Verification items for the finished model (mm, model axes). Face numbers are marked on the shaded views. A direction names the side the tool comes from. Give positions to 0.01 mm unless a question says otherwise; leave off trailing zeros. Loops run counter-clockwise (first coordinate to the right, second up) from the corner with the lowest first, then second, coordinate; pieces in that order, holes last. Notation, with made-up numbers: (-19.75, 63) -> (38.25, 63) arc R9 cw to (38.25, 68) -> close; hole circle Ø2 at (31, 22). An arc over 180 degrees is marked (long way). Answer in a Markdown table with one row per item. Add a question column.
Q1. Material ranges on probe 1 along X at (y, z) = (1, 145); probe 2 along Y at (x, z) = (11, -25.5), recorded low to high.
Q2. Section check A-A on y = 0. Enter the section's corners in (x, z) (3 decimals).
Q3. Set-up check for the marked faces 1 and 2: record each of +Z, -Z, +X, -X, +Y, -Y from which the full face is reachable in a straight line by a thin tool's end or side.
Q4. Section check B-B on x = 0. Enter the section's corners in (y, z) (3 decimals), and give its area (3 significant figures).
Q5. Gauge pin test, flat ends, axial feed: P1, Ø6, axis at y = 14.5, z = -148, coming from the -X side; P2, Ø8, axis at y = -13.5, z = 113, coming from the -X side; P3, Ø4, axis at x = 5.5, z = -72.5, coming from the -Y side. Record the tip position at first contact, or that the pin passes through.
Q6. Section check C-C on z = 109.5. Enter the section's corners in (x, y).
```python
from build123d import *

# Parameters (mm, degrees)
CUT_EXTRUDE1_REACH = 383
SKETCH4_R          = 3.175


with BuildPart() as part:
    # Sketch2 → Revolve1 (revolve)
    with BuildSketch(Plane(origin=(0, 0, 0), x_dir=(1, 0, 0), z_dir=(0, 1, 0))):
        Polygon((0, -190.5), (12.7, -190.5), (12.7, -139.7), (19.05, -133.35), (19.05, -120.65), (12.7, -114.3), (12.7, 187.325), (9.525, 190.5), (0, 190.5), align=None)
    revolve(axis=Axis((0, 0, 190.5), (0, 0, -1)))

    # Sketch4 → Cut-Extrude1 (cut, up to next)
    with BuildSketch(Plane.XY.offset(190.5), mode=Mode.PRIVATE) as cut_extrude1_sk1:
        with Locations((0, 19.05)):
            Circle(SKETCH4_R)
    cut_extrude1_tool1 = extrude(cut_extrude1_sk1.sketch, amount=-CUT_EXTRUDE1_REACH, mode=Mode.PRIVATE) & part.part
    add(cut_extrude1_tool1.solids().sort_by_distance((0, 19.05, 190.5))[0], mode=Mode.SUBTRACT)


solid = part.part
```
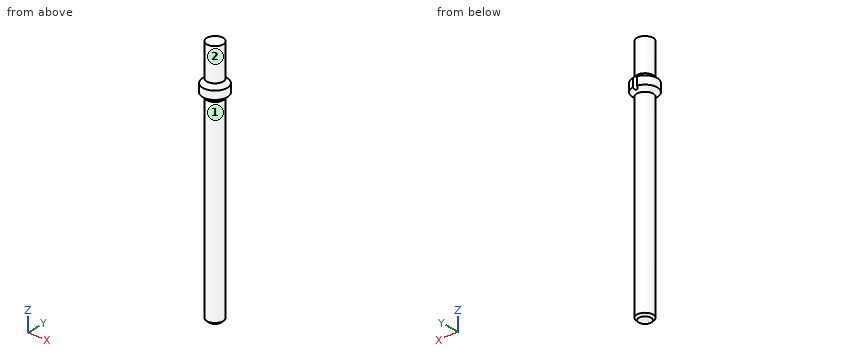
Taken from the geometry:
| question | item | result |
|---|---|---|
| 1 | probe 1 | x = -12.66 to 12.66 |
| 1 | probe 2 | y = -6.35 to 6.35 |
| 2 | outline | (-19.05, 120.65) -> (-12.7, 114.3) -> (-12.7, -187.325) -> (-9.525, -190.5) -> (9.525, -190.5) -> (12.7, -187.325) -> (12.7, 114.3) -> (19.05, 120.65) -> (19.05, 133.35) -> (12.7, 139.7) -> (12.7, 190.5) -> (-12.7, 190.5) -> (-12.7, 139.7) -> (-19.05, 133.35) -> close |
| 3 | face 1 | -Z |
| 3 | face 2 | +Z |
| 4 | outline | (-19.05, 120.65) -> (-12.7, 114.3) -> (-12.7, -187.325) -> (-9.525, -190.5) -> (9.525, -190.5) -> (12.7, -187.325) -> (12.7, 114.3) -> (15.875, 117.475) -> (15.875, 136.525) -> (12.7, 139.7) -> (12.7, 190.5) -> (-12.7, 190.5) -> (-12.7, 139.7) -> (-19.05, 133.35) -> close |
| 4 | area | 9,860 mm² |
| 5 | P1 | stops at x = -5.39 |
| 5 | P2 | stops at x = -9.48 |
| 5 | P3 | stops at y = -12.21 |
| 6 | outline | circle Ø25.4 at (0, 0) |
